Can you work these out from the drawing? Everything is in mm from the part's minimum corner. A direction names the side the tool comes from. Coordinates: 2 decimals unless noted, no trailing zeros. Write each loop counter-clockwise with the first axis right and the second up, starting at its lowest first coordinate (ties: lowest second). Pieces come first, ordered by that corner, then holes. Notation, with made-up numbers: (-25.5, 44.25) -> (5.5, 44.25) arc R20 cw to (5.5, 63.25) -> close; hole circle Ø7 at (78.5, -30). An arc over 180 degrees is marked (long way). Answer as CSV lines item,"result". Start each with the question number.
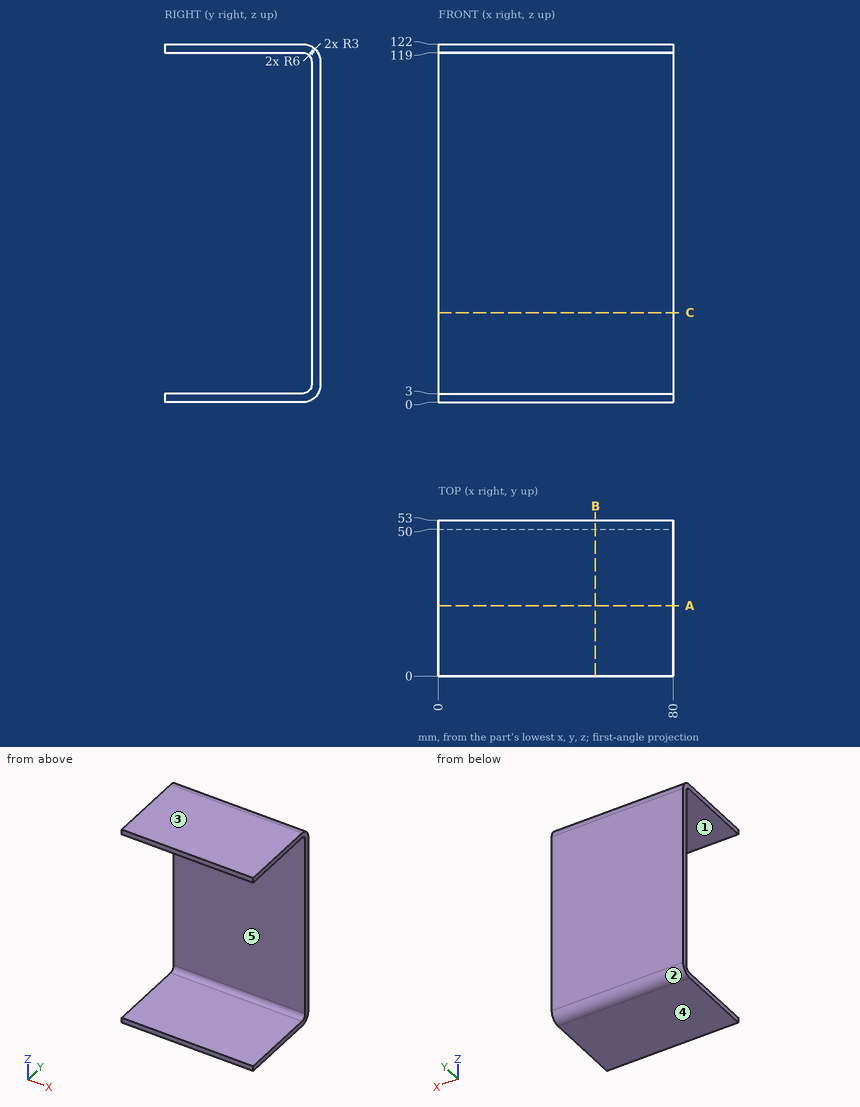
Q1. If we mould it in two halves opening along Z, with no side actions, what happens to the marked faces 1, 2 and 3? For each: released by +Z, released by -Z, zero draft, split by the parting line, or undercut.
Q2. Imagine slicing it at B-B (x = 53.5). Write out the boundary of the cut face in (y, z).
Q3. Imagine slicing it at C-C (z = 30.5). Write out the boundary of the cut face in (x, y), then the cut area to 3 significant figures.
Q4. For pin 1 (1 mm diameter, centred on x = 61, z = 17, fed in from -Y), with a flat end and sliding along its axis, tell me the tip position at first contact or that it passes through.
Q5. Imagine slicing it at A-A (y = 24). Write out the boundary of the cut face in (x, z).
Q6. Which directions (+Z, -Z, +X, -X, +Y, -Y) give clear straight access to the entire face, cutting with the end or side of a thin tool? Please do the marked faces 4 and 5.
Q7. I need wall thicknesses on L1, parallel to Z at x = 62.5, y = 45.5; L2, parallel to Y at x = 44, z = 6.5. Which ranges of each line are inside material? Lowest first, please.
Entries:
1,face 1,"undercut"
1,face 2,"released by -Z"
1,face 3,"released by +Z"
2,outline,"(0, 0) -> (47, 0) arc R6 ccw to (53, 6) -> (53, 116) arc R6 ccw to (47, 122) -> (0, 122) -> (0, 119) -> (47, 119) arc R3 cw to (50, 116) -> (50, 6) arc R3 cw to (47, 3) -> (0, 3) -> close"
3,outline,"(0, 50) -> (80, 50) -> (80, 53) -> (0, 53) -> close"
3,area,"240 mm2"
4,pin 1,"y = 50"
5,outline,"(0, 0) -> (80, 0) -> (80, 3) -> (0, 3) -> close; (0, 119) -> (80, 119) -> (80, 122) -> (0, 122) -> close"
6,face 4,"-Z, +X, -X, +Y, -Y"
6,face 5,"+X, -X, -Y"
7,L1,"0 to 3, 119 to 122"
7,L2,"50 to 53"
